from build123d import *

# Parameters (mm, degrees)
F0_R          = 25.4
F1_DEPTH      = 20
F2_W          = 25.4
F2_H          = 55.2173810765
F3_DEPTH      = 10
F4_R          = 2.54
F5_DEPTH      = 25.4
F5_DEPTH_BACK = 25.4
F6_R          = 15
F7_DEPTH      = 15


with BuildPart() as f1:
    # F0 (on Top) → F1 (new body)
    with BuildSketch(Plane.XY):
        Circle(F0_R)
    extrude(amount=F1_DEPTH)

    # F2 (on face) → F3 (cut)
    with BuildSketch(Plane.XY.offset(20)):
        with Locations((0, -0.6558205932)):
            Rectangle(F2_W, F2_H)
    extrude(amount=-F3_DEPTH, mode=Mode.SUBTRACT)

    # F4 (on Right) → F5 (cut, two sides)
    with BuildSketch(Plane.YZ) as f5_sk:
        with Locations((-12.7, 15)):
            Circle(F4_R)
        with Locations((12.7, 15)):
            Circle(F4_R)
    extrude(amount=-F5_DEPTH, mode=Mode.SUBTRACT)
    extrude(f5_sk.sketch, amount=F5_DEPTH_BACK, mode=Mode.SUBTRACT)

    # F6 (on face) → F7 (join)
    with BuildSketch(Plane.XY.offset(10)):
        Circle(F6_R)
    extrude(amount=-F7_DEPTH)


solid = f1.part
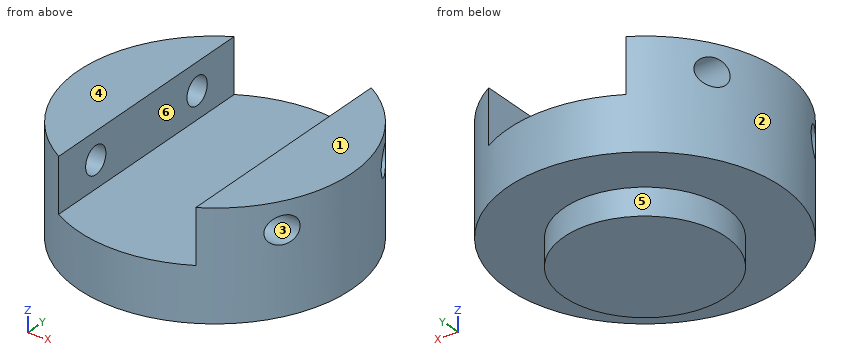
Check sheet for the modelled part. Datum: model origin and axes. Units: mm. Face numbers are marked on the shaded views. A direction names the side the tool comes from. Give positions to 0.01 mm unless a question says otherwise; leave off trailing zeros. Write each loop counter-clockwise with the first axis right and the second up, starting at its lowest first coordinate (ties: lowest second). Pieces come first, ordered by that corner, then holes. Notation, with made-up numbers: M 39,8 L 76,8 A29 ccw 76,29 Z; hole C 13.25,7.25 d2. An arc over 180 degrees is marked long. Use one line per item in the form item = value.
(1) Depth check by flat-ended pin: P1, Ø8, axis at y = 12.7, z = 15, coming from the -X side; P2, Ø5, axis at y = -20, z = 15, coming from the -X side; P3, Ø12, axis at x = 4.5, z = 4, coming from the +Y side. Enter the tip coordinate at first touch or a pass-through.
Answer block:
P1 = -23.86
P2 = -18.41
P3 = 25.4
(2) Section check C-C on x = 0. Record the boundary of the cut face in (y, z), plus the area to 3 significant figures.
Answer block:
outline = M -25.4,0 L -15,0 L -15,-5 L 15,-5 L 15,0 L 25.4,0 L 25.4,10 L -25.4,10 Z
area = 658 mm2
(3) Draft check along Y on the marked faces 1, 2 and 3. Enter one of: pulls with the +Y half, pulls with the -Y half, needs draft (parallel to the pull), parting line crosses it, or undercut.
Answer block:
face_1 = needs draft
face_2 = parting line crosses it
face_3 = undercut
(4) Material ranges on line 1 along Y through (x, z) = (19.5, 15); line 2 along Z through (x, y) = (-15.5, 12.7); line 3 along Y through (x, z) = (-15, 15), recorded low to high.
Answer block:
line_1 = -16.28 to -15.24, -10.16 to 10.16, 15.24 to 16.28
line_2 = 0 to 12.46, 17.54 to 20
line_3 = -20.5 to -15.24, -10.16 to 10.16, 15.24 to 20.5
(5) Section check B-B on y = 0. Record the boundary of the cut face in (x, z).
Answer block:
outline = M -25.4,0 L -15,0 L -15,-5 L 15,-5 L 15,0 L 25.4,0 L 25.4,20 L 12.7,20 L 12.7,10 L -12.7,10 L -12.7,20 L -25.4,20 Z
(6) Section check A-A on z = 15. Record the boundary of the cut face in (x, y).
Answer block:
outline = M -23.28,-10.16 L -12.7,-10.16 L -12.7,10.16 L -23.28,10.16 A25.4 ccw Z; M -20.32,-15.24 A25.4 ccw -12.7,-22 L -12.7,-15.24 Z; M -20.32,15.24 L -12.7,15.24 L -12.7,22 A25.4 ccw Z; M 12.7,-22 A25.4 ccw 20.32,-15.24 L 12.7,-15.24 Z; M 12.7,-10.16 L 23.28,-10.16 A25.4 ccw 23.28,10.16 L 12.7,10.16 Z; M 12.7,15.24 L 20.32,15.24 A25.4 ccw 12.7,22 Z
(7) Tool access check on the marked faces 4, 5 and 6. Record the directions out of +Z, -Z, +X, -X, +Y, -Y that give a thin tool (end or side, any length) a straight path to the whole face; none if there is none.
Answer block:
face_4 = +Z, +X, -X, +Y, -Y
face_5 = -Z
face_6 = +Z, +Y, -Y
(8) Section check D-D on y = 12.7. Record the boundary of the cut face in (x, z), plus the area to 3 significant figures.
Answer block:
outline = M -22,0 L -7.98,0 L -7.98,-5 L 7.98,-5 L 7.98,0 L 22,0 L 22,12.46 L 12.7,12.46 L 12.7,10 L -12.7,10 L -12.7,12.46 L -22,12.46 Z; M -22,17.54 L -12.7,17.54 L -12.7,20 L -22,20 Z; M 12.7,17.54 L 22,17.54 L 22,20 L 12.7,20 Z
area = 611 mm2
